Here's the drawing with two shaded views (mm, measured from the low corner). I have some questions. A direction names the side the tool comes from. Give positions to 0.01 mm unless a question says otherwise; leave off trailing zeros. Loops run counter-clockwise (first coordinate to the right, second up) from the corner with the lowest first, then second, coordinate; pieces in that order, holes last. Notation, with made-up numbers: (57.5, 29.5) -> (83.5, 29.5) arc R18 ccw to (83.5, 36.5) -> close; hole circle Ø6 at (80, 1). An arc over 180 degrees is marked (long way). Put each result on its own line as item: value.
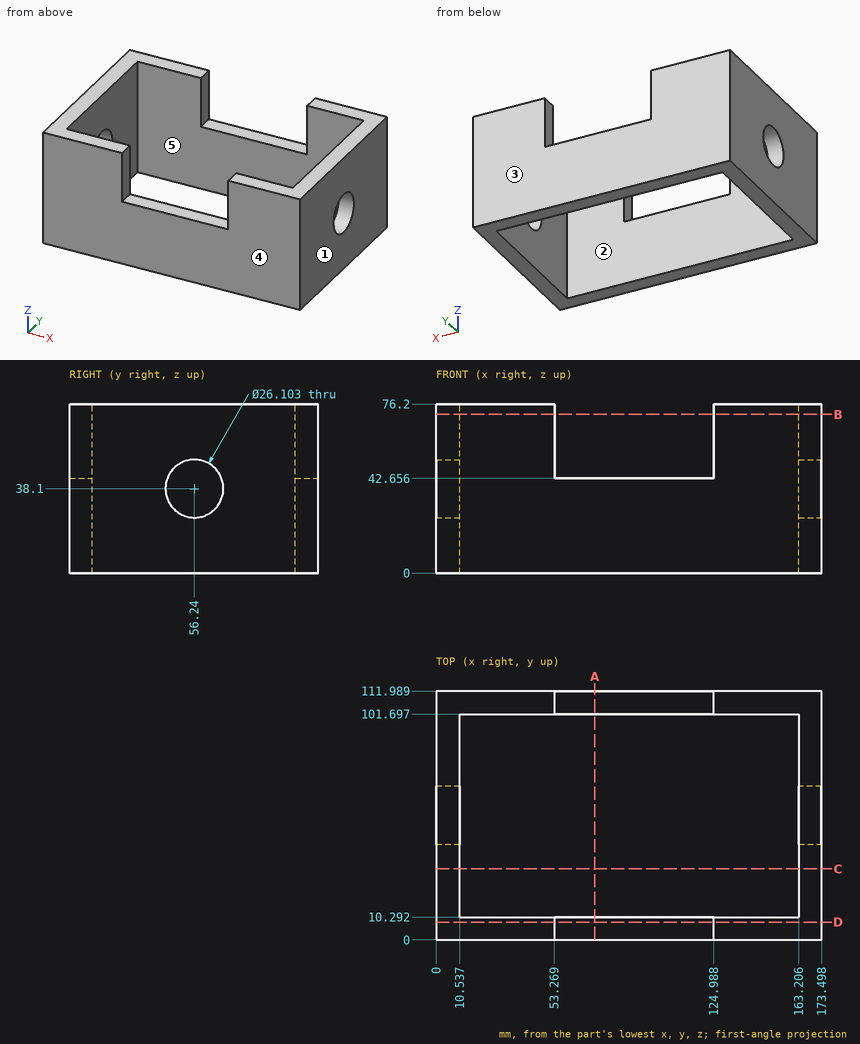
1. If we section it at A-A (x = 71.5): List the corners of the cut face in (y, z) for me (1 decimal), then the cut area to 3 significant figures.
Recorded:
outline: (0, 0) -> (10.3, 0) -> (10.3, 42.7) -> (0, 42.7) -> close; (101.7, 0) -> (112, 0) -> (112, 42.7) -> (101.7, 42.7) -> close
area: 878 mm^2
2. I'm going to push flat-ended pins straight in: pin 1 (11.5 mm diameter, centred on x = 81.5, y = 106, fed in from +Z); pin 2 (6 mm diameter, centred on x = 94.5, z = 47, fed in from +Y). Where does each tip first touch, or does it pass through?
Recorded:
pin 1: stops at z = 42.66
pin 2: passes through
3. I need wall thicknesses on line 1 (X direction, y = 103.5, z = 57.5); line 2 (X direction, y = 101, z = 6.5) (1 decimal); line 3 (Y direction, x = 170, z = 38). Which ranges of each line are inside material? Lowest first, please.
Recorded:
line 1: x = 0 to 53.27, 124.99 to 173.5
line 2: x = 0 to 10.5, 163.2 to 173.5
line 3: y = 0 to 43.19, 69.29 to 111.99
4. If we section it at C-C (y = 32): List the corners of the cut face in (x, z) for me (1 decimal).
Recorded:
outline: (0, 0) -> (10.5, 0) -> (10.5, 76.2) -> (0, 76.2) -> close; (163.2, 0) -> (173.5, 0) -> (173.5, 76.2) -> (163.2, 76.2) -> close
5. If we section it at D-D (y = 8): List the corners of the cut face in (x, z) for me (1 decimal).
Recorded:
outline: (0, 0) -> (173.5, 0) -> (173.5, 76.2) -> (125, 76.2) -> (125, 42.7) -> (53.3, 42.7) -> (53.3, 76.2) -> (0, 76.2) -> close
6. Thinking about a two-plate mould opening in X: for the marked faces 1, 2 and 3, which applies, pulls with the +X half, pulls with the -X half, needs draft (parallel to the pull), parting line crosses it, or undercut?
Recorded:
face 1: pulls with the +X half
face 2: undercut
face 3: needs draft
7. If we section it at B-B (z = 71.5): List the corners of the cut face in (x, y) for me (1 decimal).
Recorded:
outline: (0, 0) -> (53.3, 0) -> (53.3, 10.3) -> (10.5, 10.3) -> (10.5, 101.7) -> (53.3, 101.7) -> (53.3, 112) -> (0, 112) -> close; (125, 0) -> (173.5, 0) -> (173.5, 112) -> (125, 112) -> (125, 101.7) -> (163.2, 101.7) -> (163.2, 10.3) -> (125, 10.3) -> close
8. For the marked faces 4 and 5, which set-ups out of +Z, -Z, +X, -X, +Y, -Y let a thin tool reach every point of the face, with its end or its side?
Recorded:
face 4: +Z, -Z, +X, -X, -Y
face 5: +Z, -Z
